Source: three-view drawing plus pictorial views. Frame: mm from the lowest corner of the part. Give positions to 0.01 mm unless a question says otherwise; leave off trailing zeros. Order: outer loops, then holes, each group sorted by start corner. A loop starts at its lowest first (then second) coordinate and runs counter-clockwise, first axis right, second up. Notation, with made-up numbers: (-30.75, -34) -> (23.25, -34) arc R31 cw to (23.25, -8) -> close; hole circle Ø10 at (-32, 57.5). An arc over 180 degrees is marked (long way). Answer in a Markdown table with one row per item.
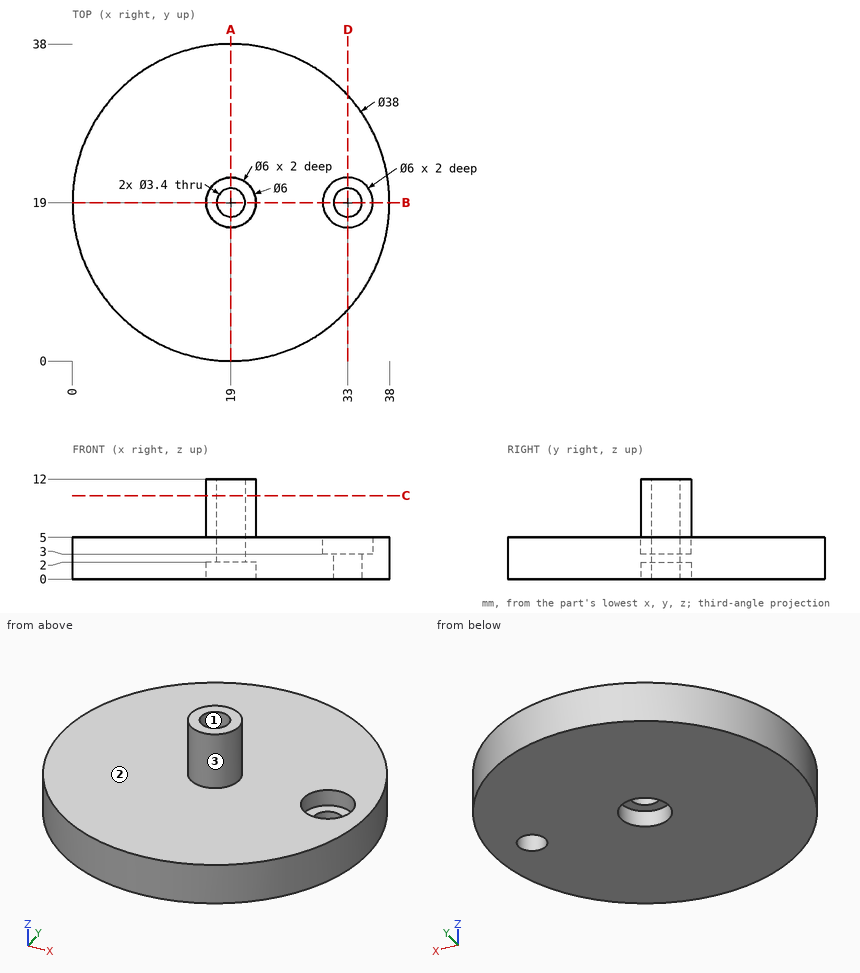
(1) First-contact query: pin 1 Ø12 at (x, y) = (29.5, 14) entering from +Z; pin 2 Ø4 at (x, y) = (19, 19) entering from -Z; pin 3 Ø6 at (y, z) = (27, 4.5) entering from +X. Flat tips, straight axial feed; report the tip coordinate or a pass-through.
A:
| item | result |
|---|---|
| pin 1 | stops at z = 5 |
| pin 2 | stops at z = 2 |
| pin 3 | stops at x = 37.33 |
(2) Ray query, probe 1 along Y at (x, z) = (19, 1.3); probe 2 along Y at (x, z) = (19, 8.5); probe 3 along Z at (x, y) = (20.5, 13). Return the intervals inside material, ascending.
A:
| item | result |
|---|---|
| probe 1 | y = 0 to 16, 22 to 38 |
| probe 2 | y = 16 to 17.3, 20.7 to 22 |
| probe 3 | z = 0 to 5 |
(3) Section query D-D (x = 33). Return the cut outline in (y, z), plus the area to 3 significant figures.
A:
| item | result |
|---|---|
| outline | (6.15, 0) -> (17.3, 0) -> (17.3, 3) -> (16, 3) -> (16, 5) -> (6.15, 5) -> close; (20.7, 0) -> (31.85, 0) -> (31.85, 5) -> (22, 5) -> (22, 3) -> (20.7, 3) -> close |
| area | 106 mm^2 |
(4) Section query B-B (y = 19). Return the cut outline in (x, z).
A:
| item | result |
|---|---|
| outline | (0, 0) -> (16, 0) -> (16, 2) -> (17.3, 2) -> (17.3, 12) -> (16, 12) -> (16, 5) -> (0, 5) -> close; (20.7, 2) -> (22, 2) -> (22, 0) -> (31.3, 0) -> (31.3, 3) -> (30, 3) -> (30, 5) -> (22, 5) -> (22, 12) -> (20.7, 12) -> close; (34.7, 0) -> (38, 0) -> (38, 5) -> (36, 5) -> (36, 3) -> (34.7, 3) -> close |
(5) Pull-direction query (X, two-part tool) for the marked faces 1, 2 and 3; classes: +X half, -X half, draft (parallel to the pull), parting line (faces both ways), or undercut.
A:
| item | result |
|---|---|
| face 1 | undercut |
| face 2 | draft |
| face 3 | parting line |
(6) Section query A-A (x = 19). Return the cut outline in (y, z), plus the area to 3 significant figures.
A:
| item | result |
|---|---|
| outline | (0, 0) -> (16, 0) -> (16, 2) -> (17.3, 2) -> (17.3, 12) -> (16, 12) -> (16, 5) -> (0, 5) -> close; (20.7, 2) -> (22, 2) -> (22, 0) -> (38, 0) -> (38, 5) -> (22, 5) -> (22, 12) -> (20.7, 12) -> close |
| area | 186 mm^2 |
(7) Section query C-C (z = 10). Return the cut outline in (x, y).
A:
| item | result |
|---|---|
| outline | circle Ø6 at (19, 19); hole circle Ø3.4 at (19, 19) |
